The model under review builds one solid part; all positions refer to its coordinate system, in mm. A direction names the side the tool comes from. Coordinates: 2 decimals unless noted, no trailing zeros. Write each loop counter-clockwise with the first axis right and the second up, starting at its lowest first coordinate (ties: lowest second). Pieces come first, ordered by that corner, then holes. Notation, with made-up numbers: M 13.5,46 L 25.5,46 A22 cw 25.5,58 Z; hole C 81,54.5 d3. An arc over 180 degrees is marked long. Answer as a JSON object with one key per item and string values.
```python
from build123d import *

# Parameters (mm, degrees)
F0_W     = 14
F0_H     = 22
F0_R     = 2
F0_H_2   = 20
F0_R_2   = 2.75
F1_DEPTH = 21
F2_DEPTH = 10
F3_R     = 4
F3_R_2   = 2
F4_DEPTH = 11
F5_R     = 2.75
F6_DEPTH = 1


with BuildPart() as f1:
    # F0 (on Front) → F1 (new body)
    with BuildSketch(Plane.XZ):
        with Locations((-7, 31)):
            Rectangle(F0_W, F0_H)
        with Locations((-7, 26)):
            Circle(F0_R, mode=Mode.SUBTRACT)
        with Locations((-7, 10)):
            Rectangle(F0_W, F0_H_2)
        with Locations((-7, 5)):
            Circle(F0_R_2, mode=Mode.SUBTRACT)
        with Locations((-7, 15)):
            Circle(F0_R_2, mode=Mode.SUBTRACT)
    extrude(amount=-F1_DEPTH)

    # F0 (on Front) → F2 (cut)
    with BuildSketch(Plane.XZ):
        with Locations((-7, 10)):
            Rectangle(F0_W, F0_H_2)
        with Locations((-7, 5)):
            Circle(F0_R_2, mode=Mode.SUBTRACT)
        with Locations((-7, 15)):
            Circle(F0_R_2, mode=Mode.SUBTRACT)
    extrude(amount=-F2_DEPTH, mode=Mode.SUBTRACT)

    # F3 (on face) → F4 (cut)
    with BuildSketch(Plane(origin=(0, 21, 0), x_dir=(-1, 0, 0), z_dir=(0, 1, 0))):
        with Locations((7, 26)):
            Circle(F3_R)
        with Locations((7, 26)):
            Circle(F3_R_2, mode=Mode.SUBTRACT)
    extrude(amount=-F4_DEPTH, mode=Mode.SUBTRACT)

    # F5 (on face) → F6 (cut)
    with BuildSketch(Plane(origin=(0, 21, 0), x_dir=(-1, 0, 0), z_dir=(0, 1, 0))):
        with BuildLine():
            Line((4, 23.354249), (4, 0))
            Line((4, 0), (10, 0))
            Line((10, 0), (10, 23.354249))
            ThreePointArc((10, 23.354249), (7, 22), (4, 23.354249))
        make_face()
        with Locations((7, 5)):
            Circle(F5_R, mode=Mode.SUBTRACT)
        with Locations((7, 15)):
            Circle(F5_R, mode=Mode.SUBTRACT)
    extrude(amount=-F6_DEPTH, mode=Mode.SUBTRACT)


solid = f1.part
```
(1) For pin 1 Ø5 at (x, z) = (-7, 15) entering from +Y; pin 2 Ø4 at (x, z) = (-8, 13.5) entering from -Y; pin 3 Ø8 at (x, y) = (-12, 3) entering from -Z; pin 4 Ø3 at (x, z) = (-7, 17.5) entering from +Y, all flat-tipped, find the tip position at first contact; note any pin that passes through.
Results list:
{"pin 1": "through", "pin 2": "y = 10", "pin 3": "z = 20", "pin 4": "y = 20"}
(2) Add section B-B on z = 25. Give the boundary of the cut face in (x, y), and give its area (3 significant figures).
Results list:
{"outline": "M -14,0 L -8.73,0 L -8.73,10 L -10.87,10 L -10.87,21 L -14,21 Z; M -5.27,0 L 0,0 L 0,21 L -3.13,21 L -3.13,10 L -5.27,10 Z", "area": "174 mm²"}
(3) Wall thickness on line 1 along Z through (x, y) = (-7, 18); line 2 along Z through (x, y) = (-7, 4); line 3 along X through (y, z) = (16.5, 26): over which ranges is each line inside the solid? List them lowest first. Write a range as from..to.
Results list:
{"line 1": "0..2.25, 7.75..12.25, 17.75..22, 30..42", "line 2": "20..24, 28..42", "line 3": "-14..-11, -3..0"}
(4) Add section C-C on x = -7. Give the boundary of the cut face in (y, z).
Results list:
{"outline": "M 0,20 L 10,20 L 10,17.75 L 20,17.75 L 20,22 L 10,22 L 10,24 L 0,24 Z; M 0,28 L 10,28 L 10,30 L 21,30 L 21,42 L 0,42 Z; M 10,0 L 20,0 L 20,2.25 L 10,2.25 Z; M 10,7.75 L 20,7.75 L 20,12.25 L 10,12.25 Z"}
(5) Add section A-A on y = 13. Give the boundary of the cut face in (x, z), and give its area (3 significant figures).
Results list:
{"outline": "M -14,0 L 0,0 L 0,42 L -14,42 Z; hole C -7,26 d8; hole C -7,5 d5.5; hole C -7,15 d5.5", "area": "490 mm²"}
(6) Add section D-D on y = 3.5. Give the boundary of the cut face in (x, z), and give its area (3 significant figures).
Results list:
{"outline": "M -14,20 L 0,20 L 0,42 L -14,42 Z; hole C -7,26 d4", "area": "295 mm²"}
(7) Draft analysis for pull direction Z (two halves, no side actions). For faces 6 (the face through (-6.479, 15.577, 29.966)), 7 (the face through (-7, 10, 42)), 8 (the face through (-7, 5, 20)), 9 (the face through (-7, 20, 12)), state which applies: released by +Z, released by -Z, zero draft, split by the parting line, or undercut.
Results list:
{"face 6": "undercut", "face 7": "released by +Z", "face 8": "released by -Z", "face 9": "zero draft"}
(8) For faces 1 (the face through (-7, 0, 31)), 2 (the face through (0, 13, 25)), 3 (the face through (-7, 10, 10)), 4 (the face through (-8, 10, 28)), 5 (the face through (-10, 20.5, 11.5)), list the 3-axis set-ups (+Z, -Z, +X, -X, +Y, -Y) from which the entire face can be reached by the end or side of a thin tool; tool diameter is ignored.
Results list:
{"face 1": "+Z, -Z, +X, -X, -Y", "face 2": "+Z, -Z, +X, +Y, -Y", "face 3": "-Z, +X, -X, -Y", "face 4": "+Y", "face 5": "-Z, +Y"}
